Input: part model. Units: mm. Frame: model coordinates. A direction names the side the tool comes from. Coordinates: 2 decimals unless noted, no trailing zeros. Order: outer loops, then holes, each group sorted by start corner. A loop starts at its lowest first (then second) coordinate and runs counter-clockwise, first axis right, second up.
from build123d import *

# Parameters (mm, degrees)
SKETCH4_W            = 31.4
SKETCH4_H            = 31.4
SKETCH4_W_2          = 25.4
SKETCH4_H_2          = 25.4
BOSS_EXTRUDE3_DEPTH  = 30
SKETCH5_W            = 31.4
SKETCH5_H            = 31.4
BOSS_EXTRUDE4_DEPTH  = 5
SKETCH6_W            = 31.4
SKETCH6_H            = 8
BOSS_EXTRUDE5_DEPTH  = 5
BOSS_EXTRUDE6_DEPTH  = 8
SKETCH8_R            = 4
BOSS_EXTRUDE7_DEPTH  = 8
SKETCH9_W            = 31.4
SKETCH9_H            = 10
BOSS_EXTRUDE8_DEPTH  = 5
SKETCH10_W           = 31.4
SKETCH10_H           = 10
BOSS_EXTRUDE9_DEPTH  = 13
SKETCH11_W           = 6.2
SKETCH11_H           = 10
BOSS_EXTRUDE10_DEPTH = 40
BOSS_EXTRUDE11_DEPTH = 3


with BuildPart() as part:
    # Sketch4 → Boss-Extrude3 (new body)
    with BuildSketch(Plane.XY):
        Rectangle(SKETCH4_W, SKETCH4_H)
        Rectangle(SKETCH4_W_2, SKETCH4_H_2, mode=Mode.SUBTRACT)
    extrude(amount=BOSS_EXTRUDE3_DEPTH)

    # Sketch5 → Boss-Extrude4 (add)
    with BuildSketch(Plane.XY.offset(30)):
        Rectangle(SKETCH5_W, SKETCH5_H)
    extrude(amount=BOSS_EXTRUDE4_DEPTH)

    # Sketch6 → Boss-Extrude5 (add)
    with BuildSketch(Plane.XY.offset(35)):
        Rectangle(SKETCH6_W, SKETCH6_H)
    extrude(amount=BOSS_EXTRUDE5_DEPTH)

    # Sketch7 → Boss-Extrude6 (add)
    with BuildSketch(Plane.XZ.offset(4)):
        with BuildLine():
            Line((-15.7, 40), (-15.7, 52))
            ThreePointArc((-15.7, 52), (-11.306601718, 62.606601718), (-0.7, 67))
            Line((-0.7, 67), (0.7, 67))
            ThreePointArc((0.7, 67), (11.306601718, 62.606601718), (15.7, 52))
            Line((15.7, 52), (15.7, 40))
            Line((15.7, 40), (-15.7, 40))
        make_face()
    extrude(amount=-BOSS_EXTRUDE6_DEPTH)

    # Sketch8 → Boss-Extrude7 (add)
    with BuildSketch(Plane.XZ.offset(4)):
        with Locations(Location((0, 52, 0), (0, 0, 180))):
            Circle(SKETCH8_R)
    boss_extrude7 = extrude(amount=BOSS_EXTRUDE7_DEPTH)

    # Mirror1: Boss-Extrude7 across plane
    add(boss_extrude7.mirror(Plane.ZX))

    # Sketch9 → Boss-Extrude8 (add)
    with BuildSketch(Plane(origin=(0, 15.7, 0), x_dir=(1, 0, 0), z_dir=(0, 1, 0))):
        with Locations((0, -27)):
            Rectangle(SKETCH9_W, SKETCH9_H)
    extrude(amount=BOSS_EXTRUDE8_DEPTH)

    # Sketch10 → Boss-Extrude9 (add)
    with BuildSketch(Plane(origin=(0, 15.7, 0), x_dir=(1, 0, 0), z_dir=(0, 1, 0))):
        with Locations((0, -17)):
            Rectangle(SKETCH10_W, SKETCH10_H)
    extrude(amount=BOSS_EXTRUDE9_DEPTH)

    # Sketch11 → Boss-Extrude10 (add)
    with BuildSketch(Plane(origin=(0, 20.7, 0), x_dir=(1, 0, 0), z_dir=(0, 1, 0))):
        with Locations((-12.6, -27)):
            Rectangle(SKETCH11_W, SKETCH11_H)
        with Locations((12.6, -27)):
            Rectangle(SKETCH11_W, SKETCH11_H)
    extrude(amount=BOSS_EXTRUDE10_DEPTH)

    # Sketch12 → Boss-Extrude11 (add)
    with BuildSketch(Plane.XY.offset(32)):
        Polygon((-15.7, 60.7), (-9.5, 60.7), (-9.5, 20.7), (9.5, 20.7), (9.5, 60.7), (15.7, 60.7), (15.7, 15.7), (-15.7, 15.7), align=None)
    extrude(amount=BOSS_EXTRUDE11_DEPTH)


solid = part.part
Item 1: Pin query (flat end, axial travel): pin 1 Ø3.5 at (x, z) = (-1.5, 5.5) entering from +Y; pin 2 Ø13 at (x, y) = (6, -11.5) entering from +Z; pin 3 Ø5 at (x, y) = (12.5, 46) entering from -Z; pin 4 Ø1 at (x, y) = (1, 30) entering from -Z. Return the tip coordinate at first contact, or that it passes through.
Response values:
pin 1: stops at y = 15.7
pin 2: stops at z = 56
pin 3: stops at z = 22
pin 4: passes through
Item 2: Access query for faces 1 (the face through (0, -10, 35)), 2 (the face through (0, 12, 52)), 3 (the face through (0, 20.7, 28)), 4 (the face through (0, 15.7, 6)). Directions: +Z, -Z, +X, -X, +Y, -Y. A direction counts if a zero-diameter tool reaches every point of the face in a straight line with its end or side. Return the directions, or none.
Response values:
face 1: +X, -X, -Y
face 2: +Z, +X, -X, +Y
face 3: +Z, +Y
face 4: -Z, +X, -X, +Y
Item 3: Cut plane D-D on y = -5.5. Return loops of the section in (x, z), then the cut area to 3 significant figures.
Response values:
outline: (-15.7, 0) - (-12.7, 0) - (-12.7, 30) - (12.7, 30) - (12.7, 0) - (15.7, 0) - (15.7, 35) - (-15.7, 35) - close; circle Ø8 at (0, 52)
area: 387 mm2
Item 4: Cut plane C-C on x = 11.5. Return loops of the section in (y, z).
Response values:
outline: (-15.7, 0) - (-12.7, 0) - (-12.7, 30) - (12.7, 30) - (12.7, 0) - (15.7, 0) - (15.7, 12) - (28.7, 12) - (28.7, 22) - (60.7, 22) - (60.7, 35) - (4, 35) - (4, 62.41) - (-4, 62.41) - (-4, 35) - (-15.7, 35) - close
Item 5: Ray query, probe 1 along Y at (x, z) = (-10, 4.5); probe 2 along X at (y, z) = (48.5, 28). Return the intervals inside material, ascending.
Response values:
probe 1: y = -15.7 to -12.7, 12.7 to 15.7
probe 2: x = -15.7 to -9.5, 9.5 to 15.7
Item 6: Draft query along Z for faces 5 (the face through (0, 22, 12)), 6 (the face through (-1.846, 7.944, 55.549)), 7 (the face through (0, 28.7, 17)). Return one class per face: pulls with the +Z half, pulls with the -Z half, needs draft (parallel to the pull), parting line crosses it, or undercut.
Response values:
face 5: pulls with the -Z half
face 6: undercut
face 7: needs draft
Item 7: Cut plane B-B on z = 16. Return loops of the section in (x, y), then the cut area to 3 significant figures.
Response values:
outline: (-15.7, -15.7) - (15.7, -15.7) - (15.7, 28.7) - (-15.7, 28.7) - close; hole (-12.7, -12.7) - (12.7, -12.7) - (12.7, 12.7) - (-12.7, 12.7) - close
area: 749 mm2
Item 8: Cut plane A-A on y = 32. Return loops of the section in (x, z).
Response values:
outline: (-15.7, 22) - (-9.5, 22) - (-9.5, 35) - (-15.7, 35) - close; (9.5, 22) - (15.7, 22) - (15.7, 35) - (9.5, 35) - close
